Study the drawing (mm; zero at the part's minimum x, y, z) and answer. A direction names the side the tool comes from. Round coordinates to 2 decimals unless told otherwise and drop trailing zeros. Write each loop counter-clockwise with the first axis right and the second up, starting at its lowest first coordinate (ties: lowest second). Pieces come first, ordered by that corner, then holes.
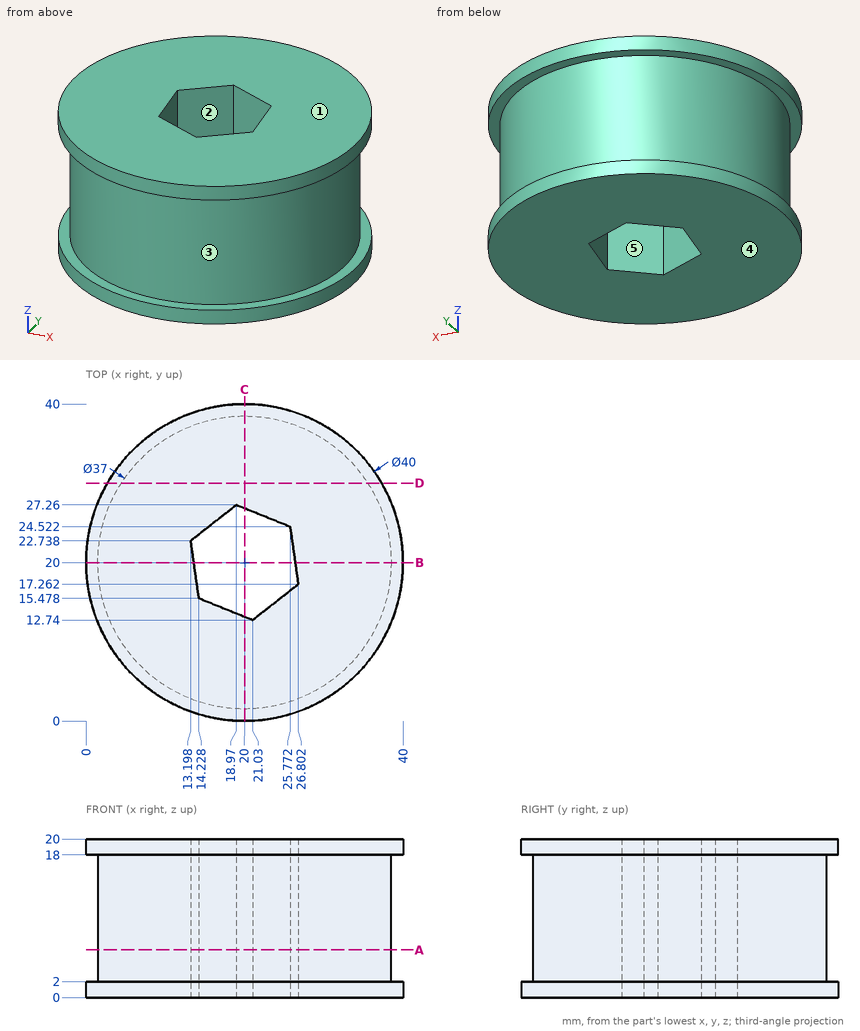
1. For a pull along Y with two mould halves and no side action, classify the marked faces 3, 4 and 5 as released by +Y, released by -Y, zero draft, split by the parting line, or undercut.
Geometry says:
face 3: split by the parting line
face 4: zero draft
face 5: undercut
2. Section C-C on x = 20 is taken. Determine the outline of the cut face in (y, z) (1 decimal).
Geometry says:
outline: (0, 0) - (13.2, 0) - (13.2, 20) - (0, 20) - (0, 18) - (1.5, 18) - (1.5, 2) - (0, 2) - close; (26.8, 0) - (40, 0) - (40, 2) - (38.5, 2) - (38.5, 18) - (40, 18) - (40, 20) - (26.8, 20) - close
3. Straight lines are drawn through the part: line 1 along Z through (x, y) = (5, 32.5); line 2 along X through (y, z) = (23, 11) (1 decimal); line 3 along Y through (x, z) = (17.5, 5). For each, find the intervals that lie inside material, in ascending order.
Geometry says:
line 1: z = 0 to 2, 18 to 20
line 2: x = 1.7 to 13.5, 26 to 38.3
line 3: y = 1.67 to 14.16, 26.11 to 38.33
4. Given pin 1 (10 mm diameter, centred on x = 26.5, z = 8, fed in from +Y); pin 2 (10 mm diameter, centred on x = 10, z = 6.5, fed in from -Y); pin 3 (1.5 mm diameter, centred on x = 10.5, z = 10.5, fed in from +Y), each flat-ended and moving along its own axis, determine where each tip first touches the part or whether it passes through.
Geometry says:
pin 1: stops at y = 38.44
pin 2: stops at y = 1.59
pin 3: stops at y = 36.3
5. Section B-B on y = 20 is taken. Determine the outline of the cut face in (x, z).
Geometry says:
outline: (0, 0) - (13.59, 0) - (13.59, 20) - (0, 20) - (0, 18) - (1.5, 18) - (1.5, 2) - (0, 2) - close; (26.41, 0) - (40, 0) - (40, 2) - (38.5, 2) - (38.5, 18) - (40, 18) - (40, 20) - (26.41, 20) - close
6. Section A-A on z = 6 is taken. Determine the outline of the cut face in (x, y).
Geometry says:
outline: circle Ø37 at (20, 20); hole (13.2, 22.74) - (14.23, 15.48) - (21.03, 12.74) - (26.8, 17.26) - (25.77, 24.52) - (18.97, 27.26) - close
7. A tool of negligible diameter and unlimited length cuts with its end or side. For the marked faces 1 and 2, from which of +Z, -Z, +X, -X, +Y, -Y can it reach the whole face along a straight path? Write none if from no direction.
Geometry says:
face 1: +Z, +X, -X, +Y, -Y
face 2: +Z, -Z
8. Section D-D on y = 30 is taken. Determine the outline of the cut face in (x, z) (1 decimal), plus the area to 3 significant figures.
Geometry says:
outline: (2.7, 0) - (37.3, 0) - (37.3, 2) - (35.6, 2) - (35.6, 18) - (37.3, 18) - (37.3, 20) - (2.7, 20) - (2.7, 18) - (4.4, 18) - (4.4, 2) - (2.7, 2) - close
area: 637 mm2
